Geometry check sheet. Reference: drawing and pictorial views, mm from the part's lowest x, y, z. A direction names the side the tool comes from. Coordinates: 2 decimals unless noted, no trailing zeros. Loops run counter-clockwise (first coordinate to the right, second up) from the corner with the lowest first, then second, coordinate; pieces in that order, holes last. Notation, with made-up numbers: (50, 24.25) - (87, 24.25) arc R3 ccw to (87, 28.25) - close; hole circle Ø7 at (86, -17.75). An arc over 180 degrees is marked (long way). Use a Markdown table: item, result. Add a question column.
1) Sectioned sample at D-D, the plane x = 45. Enter the section's corners in (y, z), then the cut area to 3 significant figures.
2) Thickness scan on line 1 (Z direction, x = 35.5, y = 9); line 2 (X direction, y = 2, z = 57); line 3 (X direction, y = 8, z = 5.5). Record the ranges inside material, lowest first.
3) Tool access check on the marked faces 4 and 5. Record the directions out of +Z, -Z, +X, -X, +Y, -Y that give a thin tool (end or side, any length) a straight path to the whole face; none if there is none.
4) Draft check along X on the marked faces 1, 2 and 3. Enter one of: pulls with the +X half, pulls with the -X half, needs draft (parallel to the pull), parting line crosses it, or undercut.
5) Sectioned sample at A-A, the plane y = 8.25. Enter the section's corners in (x, z).
6) Go/stop test with flat-tipped pins: P1, Ø4, axis at x = 46.5, z = 39, coming from the +Y side; P2, Ø1.6, axis at x = 63.5, z = 33, coming from the +Y side; P3, Ø2.5, axis at x = 4.5, y = 12, coming from the -Z side. Record where each tip stops, or that it passes through.
7) Sectioned sample at C-C, the plane x = 11.5. Enter the section's corners in (y, z).
8) Sectioned sample at B-B, the plane z = 56. Enter the section's corners in (x, y).
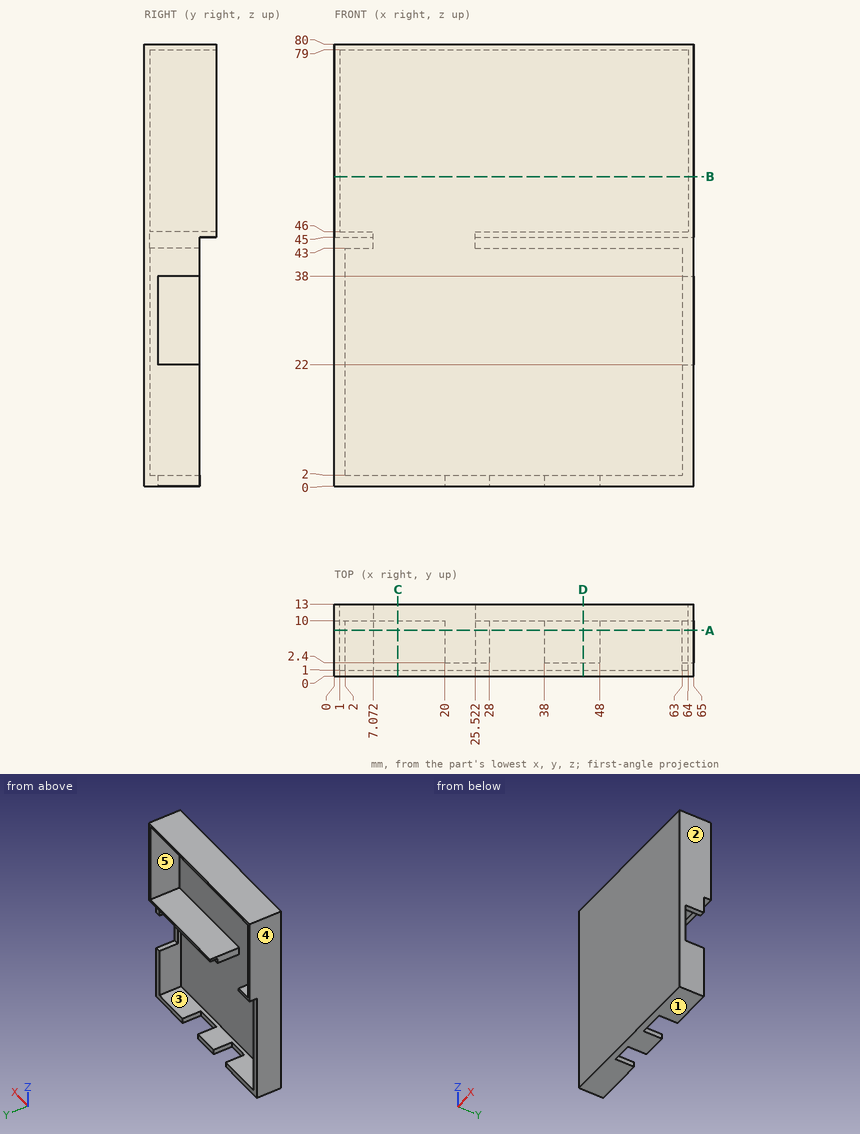
Solved:
| question | item | result |
|---|---|---|
| 1 | outline | (0, 0) - (2.4, 0) - (2.4, 2) - (1, 2) - (1, 43) - (10, 43) - (10, 45) - (13, 45) - (13, 46) - (1, 46) - (1, 79) - (13, 79) - (13, 80) - (0, 80) - close |
| 1 | area | 125 mm2 |
| 2 | line 1 | z = 0 to 2, 43 to 46, 79 to 80 |
| 2 | line 2 | x = 0 to 1, 64 to 65 |
| 2 | line 3 | x = 0 to 2, 63 to 65 |
| 3 | face 4 | +Z, -Z, -X, +Y, -Y |
| 3 | face 5 | +Y |
| 4 | face 1 | needs draft |
| 4 | face 2 | pulls with the +X half |
| 4 | face 3 | undercut |
| 5 | outline | (0, 0) - (20, 0) - (20, 2) - (2, 2) - (2, 43) - (7.07, 43) - (7.07, 46) - (1, 46) - (1, 79) - (64, 79) - (64, 46) - (25.52, 46) - (25.52, 43) - (63, 43) - (63, 38) - (65, 38) - (65, 80) - (0, 80) - close; (28, 0) - (38, 0) - (38, 2) - (28, 2) - close; (48, 0) - (65, 0) - (65, 22) - (63, 22) - (63, 2) - (48, 2) - close |
| 6 | P1 | stops at y = 1 |
| 6 | P2 | stops at y = 2.4 |
| 6 | P3 | stops at z = 45 |
| 7 | outline | (0, 0) - (10, 0) - (10, 2) - (1, 2) - (1, 79) - (13, 79) - (13, 80) - (0, 80) - close |
| 8 | outline | (0, 0) - (65, 0) - (65, 13) - (64, 13) - (64, 1) - (1, 1) - (1, 13) - (0, 13) - close |
